Input: part model. Units: mm. Frame: model coordinates. A direction names the side the tool comes from. Give positions to 0.01 mm unless a question says otherwise; leave off trailing zeros. Write each loop counter-clockwise with the first axis right and the second up, starting at its lowest first coordinate (ties: lowest second). Pieces come first, ordered by that corner, then holes. Notation, with made-up numbers: (77.25, -23.75) - (130.25, -23.75) arc R25 cw to (130.25, 3.25) - close; hole circle Ø10 at (73.25, 35.5). An arc over 180 degrees is marked (long way). Use a Markdown table: item, result. Add a question column.
1. Pin query (flat end, axial travel): pin 1 (8 mm diameter, centred on y = -7, z = 0, fed in from -X); pin 2 (1.3 mm diameter, centred on x = 5.5, y = -8.5, fed in from -Z); pin 3 (1 mm diameter, centred on x = 5.5, y = 0.5, fed in from +Z). Return the tip coordinate at first contact, or that it passes through.
2. Section query C-C, the plane z = 0. Return loops of the section in (x, y).
3. Material intervals for probe 1 along X at (y, z) = (-11.25, 1.5); probe 2 along Y at (x, z) = (3, -4.5); probe 3 along Z at (x, y) = (-2, 0.75), sorted ascending.
4. Section query D-D, the plane x = 0. Return loops of the section in (y, z), plus the area to 3 significant figures.
5. Section query A-A, the plane z = -3.6. Return loops of the section in (x, y), plus the area to 3 significant figures.
6. Section query B-B, the plane y = -3.35. Return loops of the section in (x, z), plus the area to 3 significant figures.
7. Mould query, pull axis X, two halves, no side actions, for faces 6 (the flat face through (5, -8, 0)), 7 (the cylindrical face through (5.6, -12.4, 11)), 8 (the cylindrical face through (0.03, 0.35, 2.85)). Classes: released by +X, released by -X, zero draft, split by the parting line, or undercut.
8. Set-up query: faces 1 (the flat face through (6, -16, -8)), 2 (the flat face through (0, 1, 6)), 3 (the flat face through (6, 0, 8)), 4 (the flat face through (1, 1, -6)), 5 (the flat face through (6, 0, -8)). Return all of +Z, -Z, +X, -X, +Y, -Y with unobstructed straight access to the full face (end or side cutting, diameter ignored); none if empty.
```python
from build123d import *

# Parameters (mm, degrees)
SKETCH1_R           = 0.75
SKETCH1_R_2         = 2.5
BOSS_EXTRUDE3_DEPTH = 1.2
FILLET10_R          = 1
FILLET11_R          = 1
BOSS_EXTRUDE5_DEPTH = 1.2
SKETCH6_R           = 1.25
CUT_EXTRUDE3_DEPTH  = 1.2
SKETCH7_R           = 1.25
CUT_EXTRUDE4_DEPTH  = 1.2
CHAMFER5_SIZE       = 0.5
CHAMFER6_SIZE       = 0.5
FILLET13_R          = 0.5
FILLET14_R          = 0.2
CHAMFER7_SIZE       = 0.5
CHAMFER8_SIZE       = 0.5


with BuildPart() as part:
    # Sketch1 → Boss-Extrude3 (new body)
    with BuildSketch(Plane(origin=(0, 0, 0), x_dir=(1, 0, 0), z_dir=(0, 1, 0))):
        Polygon((5, 6), (0, 6), (-5, 6), (-5, -6), (5, -6), align=None)
        with Locations(Location((0, -3.6, 0), (0, 0, 270))):
            Circle(SKETCH1_R, mode=Mode.SUBTRACT)
        with Locations(Location((0, 0, 0), (0, 0, 270))):
            Circle(SKETCH1_R_2, mode=Mode.SUBTRACT)
        with Locations(Location((0, 3.6, 0), (0, 0, 270))):
            Circle(SKETCH1_R, mode=Mode.SUBTRACT)
    extrude(amount=BOSS_EXTRUDE3_DEPTH)

    # Fillet10
    fillet10_edges = [part.edges().sort_by_distance(p)[0] for p in [
        (-5, 0.6, 6),
    ]]
    fillet(fillet10_edges, radius=FILLET10_R)

    # Fillet11
    fillet11_edges = [part.edges().sort_by_distance(p)[0] for p in [
        (-5, 0.6, -6),
    ]]
    fillet(fillet11_edges, radius=FILLET11_R)

    # Sketch5 → Boss-Extrude5 (add)
    with BuildSketch(Plane(origin=(5, 0, 0), x_dir=(0, 0, -1), z_dir=(1, 0, 0))):
        with BuildLine():
            Line((6, 1.2), (-6, 1.2))
            Line((-6, 1.2), (-8, 1.2))
            Line((-8, 1.2), (-8, -0.35))
            ThreePointArc((-8, -0.35), (-11, -3.35), (-8, -6.35))
            Line((-8, -6.35), (-8, -9.45))
            ThreePointArc((-8, -9.45), (-11, -12.45), (-8, -15.45))
            Line((-8, -15.45), (-8, -17))
            Line((-8, -17), (8, -17))
            Line((8, -17), (8, -15.45))
            ThreePointArc((8, -15.45), (11, -12.45), (8, -9.45))
            Line((8, -9.45), (8, -6.35))
            ThreePointArc((8, -6.35), (11, -3.35), (8, -0.35))
            Line((8, -0.35), (8, 1.2))
            Line((8, 1.2), (6, 1.2))
        make_face()
    extrude(amount=BOSS_EXTRUDE5_DEPTH)

    # Sketch6 → Cut-Extrude3 (cut)
    with BuildSketch(Plane(origin=(6.2, 0, 0), x_dir=(0, 0, -1), z_dir=(1, 0, 0))):
        with Locations((8, -3.35)):
            Circle(SKETCH6_R)
        with Locations((8, -12.45)):
            Circle(SKETCH6_R)
    extrude(amount=-CUT_EXTRUDE3_DEPTH, mode=Mode.SUBTRACT)

    # Sketch7 → Cut-Extrude4 (cut)
    with BuildSketch(Plane.ZY.offset(-5)):
        with Locations((8, -12.45)):
            Circle(SKETCH7_R)
        with Locations((8, -3.35)):
            Circle(SKETCH7_R)
    extrude(amount=-CUT_EXTRUDE4_DEPTH, mode=Mode.SUBTRACT)

    # Chamfer5
    chamfer5_edges = [part.edges().sort_by_distance(p)[0] for p in [
        (5, -3.35, 6.75),
    ]]
    chamfer(chamfer5_edges, length=CHAMFER5_SIZE)

    # Chamfer6
    chamfer6_edges = [part.edges().sort_by_distance(p)[0] for p in [
        (5, -3.35, -6.75),
        (5, -12.45, -6.75),
        (5, -12.45, 6.75),
    ]]
    chamfer(chamfer6_edges, length=CHAMFER6_SIZE)

    # Fillet13
    # the kernel refuses this fillet: 0.5 mm, written as the material it takes off along each edge
    with BuildSketch(Plane(origin=(0, 0, 0), x_dir=(0, 0, 1), z_dir=(-1, 0, 0))) as fillet13_piece_1:
        with BuildLine():
            CenterArc((2.5 + FILLET13_R, FILLET13_R), FILLET13_R, 180, 90)
            Line((2.5, FILLET13_R), (2.5, 0))
            Line((2.5, 0), (2.5 + FILLET13_R, 0))
        make_face()
    revolve(axis=Axis((0, 0, 0), (0, 1, 0)), mode=Mode.SUBTRACT)

    # Fillet14
    fillet14_edges = [part.edges().sort_by_distance(p)[0] for p in [
        (0, 1.2, -2.5),
    ]]
    fillet(fillet14_edges, radius=FILLET14_R)

    # Chamfer7
    # the kernel refuses this chamfer: 0.5 mm, written as the material it takes off along each edge
    with BuildSketch(Plane(origin=(0, 1.2, 3.6), x_dir=(0, 0, 1), z_dir=(-1, 0, 0))) as chamfer7_piece_1:
        Polygon((0.75 + CHAMFER7_SIZE, 0), (0.75, -CHAMFER7_SIZE), (0.75, 0), align=None)
    revolve(axis=Axis((0, 1.2, 3.6), (0, 1, 0)), mode=Mode.SUBTRACT)

    # Chamfer8
    # the kernel refuses this chamfer: 0.5 mm, written as the material it takes off along each edge
    with BuildSketch(Plane(origin=(0, 1.2, -3.6), x_dir=(0, 0, 1), z_dir=(-1, 0, 0))) as chamfer8_piece_1:
        Polygon((0.75 + CHAMFER8_SIZE, 0), (0.75, -CHAMFER8_SIZE), (0.75, 0), align=None)
    revolve(axis=Axis((0, 1.2, -3.6), (0, 1, 0)), mode=Mode.SUBTRACT)


solid = part.part
```
Result sheet:
| question | item | result |
|---|---|---|
| 1 | pin 1 | stops at x = 5 |
| 1 | pin 2 | stops at z = -8 |
| 1 | pin 3 | stops at z = 8 |
| 2 | outline | (-5, 0) - (-3, 0) arc R0.5 ccw to (-2.5, 0.5) - (-2.5, 1) arc R0.2 ccw to (-2.7, 1.2) - (-5, 1.2) - close; (2.5, 0.5) arc R0.5 ccw to (3, 0) - (5, 0) - (5, -17) - (6.2, -17) - (6.2, 1.2) - (2.7, 1.2) arc R0.2 ccw to (2.5, 1) - close |
| 3 | probe 1 | x = 5 to 6.2 |
| 3 | probe 2 | y = 0 to 1.2 |
| 3 | probe 3 | z = -6 to -1.5, 1.5 to 6 |
| 4 | outline | (0, -6) - (1.2, -6) - (1.2, -4.85) - (0.7, -4.35) - (0, -4.35) - close; (0, 4.35) - (0.7, 4.35) - (1.2, 4.85) - (1.2, 6) - (0, 6) - close; (0.02, -2.85) - (0.7, -2.85) - (1.04, -2.51) arc R0.2 ccw to (1, -2.5) - (0.5, -2.5) arc R0.5 ccw to start; (0.02, 2.85) arc R0.5 ccw to (0.5, 2.5) - (1, 2.5) arc R0.2 ccw to (1.04, 2.51) - (0.7, 2.85) - close |
| 4 | area | 4.22 mm² |
| 5 | outline | (-5, 0) - (-0.75, 0) - (-0.75, 0.7) - (-1.25, 1.2) - (-5, 1.2) - close; (0.75, 0) - (5, 0) - (5, -17) - (6.2, -17) - (6.2, 1.2) - (1.25, 1.2) - (0.75, 0.7) - close |
| 5 | area | 31.8 mm² |
| 6 | outline | (5, -11) - (6.2, -11) - (6.2, -9.25) - (5.5, -9.25) - (5, -9.75) - close; (5, -6.25) - (5.5, -6.75) - (6.2, -6.75) - (6.2, 6.75) - (5.5, 6.75) - (5, 6.25) - close; (5, 9.75) - (5.5, 9.25) - (6.2, 9.25) - (6.2, 11) - (5, 11) - close |
| 6 | area | 19.9 mm² |
| 7 | face 6 | released by -X |
| 7 | face 7 | zero draft |
| 7 | face 8 | undercut |
| 8 | face 1 | -Z, +X, -X, -Y |
| 8 | face 2 | +Z, -X, +Y, -Y |
| 8 | face 3 | +Z, +X, -X, +Y |
| 8 | face 4 | -Z, -X, +Y, -Y |
| 8 | face 5 | -Z, +X, -X, +Y |
